Part model, mm, in its own coordinate system. Coordinates: 2 decimals unless noted, no trailing zeros. Order: outer loops, then holes, each group sorted by start corner. A loop starts at its lowest first (then second) coordinate and runs counter-clockwise, first axis right, second up.
from build123d import *

# Parameters (mm, degrees)
SKETCH1_W           = 22.6
SKETCH1_H           = 70.5
BOSS_EXTRUDE1_DEPTH = 2
SKETCH2_W           = 22.6
SKETCH2_H           = 2
BOSS_EXTRUDE2_DEPTH = 22.6
SKETCH3_W           = 2
SKETCH3_H           = 9.9
SKETCH3_W_2         = 9.9
SKETCH3_H_2         = 2
BOSS_EXTRUDE3_DEPTH = 2
SKETCH4_W           = 2
SKETCH4_H           = 9.9
BOSS_EXTRUDE4_DEPTH = 2
FILLET1_R           = 2
SKETCH5_W           = 5
SKETCH5_H           = 2
BOSS_EXTRUDE5_DEPTH = 11.1
FILLET2_R           = 2
SKETCH6_R           = 3.65
SKETCH6_R_2         = 1.95
CUT_EXTRUDE1_DEPTH  = 2


with BuildPart() as part:
    # Sketch1 → Boss-Extrude1 (new body)
    with BuildSketch(Plane.XY):
        Rectangle(SKETCH1_W, SKETCH1_H)
    extrude(amount=BOSS_EXTRUDE1_DEPTH)

    # Sketch2 → Boss-Extrude2 (add)
    with BuildSketch(Plane.XY.offset(2)):
        with Locations((0, 34.25)):
            Rectangle(SKETCH2_W, SKETCH2_H)
    extrude(amount=BOSS_EXTRUDE2_DEPTH)

    # Sketch3 → Boss-Extrude3 (add)
    with BuildSketch(Plane(origin=(0, 35.25, 0), x_dir=(1, 0, 0), z_dir=(0, 1, 0))):
        with Locations((-12.3, -12.3)):
            Rectangle(SKETCH3_W, SKETCH3_H)
        with Locations((12.3, -12.3)):
            Rectangle(SKETCH3_W, SKETCH3_H)
        with Locations((0, -25.6)):
            Rectangle(SKETCH3_W_2, SKETCH3_H_2)
    extrude(amount=-BOSS_EXTRUDE3_DEPTH)

    # Sketch4 → Boss-Extrude4 (add)
    with BuildSketch(Plane.XY.offset(2)):
        with Locations((12.3, 11.75)):
            Rectangle(SKETCH4_W, SKETCH4_H)
        with Locations((12.3, -11.75)):
            Rectangle(SKETCH4_W, SKETCH4_H)
        with Locations((-12.3, -11.75)):
            Rectangle(SKETCH4_W, SKETCH4_H)
        with Locations((-12.3, 11.75)):
            Rectangle(SKETCH4_W, SKETCH4_H)
    extrude(amount=-BOSS_EXTRUDE4_DEPTH)

    # Fillet1
    # the kernel refuses this fillet: 2 mm, written as the material it takes off along each edge
    with BuildSketch(Plane(origin=(16.3, 35.25, 0), x_dir=(0, -1, 0), z_dir=(-1, 0, 0))) as fillet1_piece_1:
        with BuildLine():
            CenterArc((FILLET1_R, FILLET1_R), FILLET1_R, 180, 90)
            Line((0, FILLET1_R), (0, 0))
            Line((0, 0), (FILLET1_R, 0))
        make_face()
    extrude(amount=32.6, mode=Mode.SUBTRACT)
    with BuildSketch(Plane(origin=(13.3, 35.25, 2.35), x_dir=(-1, 0, 0), z_dir=(0, 0, 1)), Plane(origin=(9.95, 35.25, 26.6), x_dir=(0, 0, -1), z_dir=(-1, 0, 0)), Plane(origin=(-13.3, 35.25, 22.25), x_dir=(1, 0, 0), z_dir=(0, 0, -1)), Plane(origin=(13.3, 1.8, 0), x_dir=(-1, 0, 0), z_dir=(0, 1, 0)), Plane(origin=(13.3, -21.7, 0), x_dir=(-1, 0, 0), z_dir=(0, 1, 0))) as fillet1_piece_2:
        with BuildLine():
            CenterArc((FILLET1_R, FILLET1_R), FILLET1_R, 180, 90)
            Line((0, FILLET1_R), (0, 0))
            Line((0, 0), (FILLET1_R, 0))
        make_face()
    extrude(amount=19.9, mode=Mode.SUBTRACT)
    with BuildSketch(Plane(origin=(-13.3, -21.7, 0), x_dir=(1, 0, 0), z_dir=(0, 1, 0)), Plane(origin=(-13.3, 1.8, 0), x_dir=(1, 0, 0), z_dir=(0, 1, 0))) as fillet1_piece_3:
        with BuildLine():
            CenterArc((FILLET1_R, -FILLET1_R), FILLET1_R, 90, 90)
            Line((0, -FILLET1_R), (0, 0))
            Line((0, 0), (FILLET1_R, 0))
        make_face()
    extrude(amount=19.9, mode=Mode.SUBTRACT)

    # Sketch5 → Boss-Extrude5 (add)
    with BuildSketch(Plane(origin=(0, 0, 0), x_dir=(-1, 0, 0), z_dir=(0, 0, -1))):
        with Locations((0, -36.25)):
            Rectangle(SKETCH5_W, SKETCH5_H)
    extrude(amount=-BOSS_EXTRUDE5_DEPTH)

    # Fillet2
    fillet2_edges = [part.edges().sort_by_distance(p)[0] for p in [
        (0, -37.25, 0),
    ]]
    fillet(fillet2_edges, radius=FILLET2_R)

    # Sketch6 → Cut-Extrude1 (cut)
    with BuildSketch(Plane(origin=(0, 0, 0), x_dir=(-1, 0, 0), z_dir=(0, 0, -1))):
        with Locations((0, -24.05)):
            Circle(SKETCH6_R)
        with Locations((0, -12.75)):
            Circle(SKETCH6_R_2)
    extrude(amount=-CUT_EXTRUDE1_DEPTH, mode=Mode.SUBTRACT)


solid = part.part
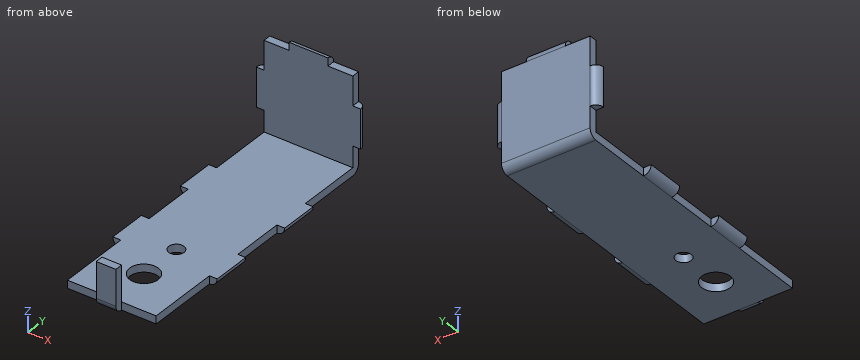
Q1. Cut at B-B on y = -24.05. Write the cut outline in (x, z), and give its area (3 significant figures).
Results list:
outline: (-11.3, 0) - (-3.65, 0) - (-3.65, 2) - (-11.3, 2) - close; (3.65, 0) - (11.3, 0) - (11.3, 2) - (3.65, 2) - close
area: 30.6 mm2
Q2. Cut at C-C on z = 6. Write the cut outline in (x, y), and give its area (3 significant figures).
Results list:
outline: (-11.3, 33.25) - (11.3, 33.25) - (11.3, 35.25) - (-11.3, 35.25) - close; (-2.5, -37.25) - (2.5, -37.25) - (2.5, -35.25) - (-2.5, -35.25) - close
area: 55.2 mm2
Q3. Wall check: line 1 along Y through (x, z) = (0, 1.45); line 2 along Y through (x, z) = (0, 1.05); line 3 along Z through (x, y) = (-6, 32). Give the ranges that are in metal, low to high.
Results list:
line 1: y = -37.17 to -27.7, -20.4 to -14.7, -10.8 to 35.17
line 2: y = -37.01 to -27.7, -20.4 to -14.7, -10.8 to 35.01
line 3: z = 0 to 2
Q4. Cut at A-A on x = 0. Write the cut outline in (y, z), and give its area (3 significant figures).
Results list:
outline: (-37.25, 2) arc R2 ccw to (-35.25, 0) - (-27.7, 0) - (-27.7, 2) - (-35.25, 2) - (-35.25, 11.1) - (-37.25, 11.1) - close; (-20.4, 0) - (-14.7, 0) - (-14.7, 2) - (-20.4, 2) - close; (-10.8, 0) - (33.25, 0) arc R2 ccw to (35.25, 2) - (35.25, 24.6) arc R2 ccw to (33.25, 26.6) - (33.25, 2) - (-10.8, 2) - close
area: 187 mm2
Q5. Cut at D-D on x = -8.25. Write the cut outline in (y, z).
Results list:
outline: (-35.25, 0) - (33.25, 0) arc R2 ccw to (35.25, 2) - (35.25, 24.6) - (33.25, 24.6) - (33.25, 2) - (-35.25, 2) - close
Q6. Pin check, flat tips, straight feed: pin 1 Ø1.6 at (x, z) = (12, 0.5) entering from -Y; pin 2 Ø8 at (x, y) = (9, 8.5) entering from +Z; pin 3 Ø2 at (x, z) = (12.5, 1) entering from -Y. Stop position of each tip, or through.
Results list:
pin 1: stops at y = -35.25
pin 2: stops at z = 2
pin 3: stops at y = -16.7
